from build123d import *

# Parameters (mm, degrees)
SKETCH1_R           = 5
BOSS_EXTRUDE1_DEPTH = 3


with BuildPart() as part:
    # Sketch1 → Boss-Extrude1 (new body)
    with BuildSketch(Plane(origin=(0, 0, 0), x_dir=(1, 0, 0), z_dir=(0, 1, 0))):
        Polygon((3, 10), (0, 10), (0, 0), (4, 0), (4, 3), (14, 3), (14, 0), (22, 0), (22, 3), (28, 3), (28, 0), (36, 0), (36, 3), (46, 3), (46, 0), (50, 0), (50, 10), (47, 10), (47, 20), (50, 20), (50, 30), (47, 30), (47, 40), (50, 40), (50, 50), (47, 50), (47, 60), (50, 60), (50, 70), (47, 70), (47, 80), (50, 80), (50, 90), (47, 90), (47, 100), (50, 100), (50, 110), (47, 110), (47, 120), (3, 120), (3, 110), (0, 110), (0, 100), (3, 100), (3, 90), (0, 90), (0, 80), (3, 80), (3, 70), (0, 70), (0, 60), (3, 60), (3, 50), (0, 50), (0, 40), (3, 40), (3, 30), (0, 30), (0, 20), (3, 20), align=None)
        with Locations(Location((25, 40, 0), (0, 0, 270))):
            Circle(SKETCH1_R, mode=Mode.SUBTRACT)
        with Locations(Location((25, 80, 0), (0, 0, 270))):
            Circle(SKETCH1_R, mode=Mode.SUBTRACT)
    extrude(amount=BOSS_EXTRUDE1_DEPTH)


solid = part.part
Geometry check sheet. Reference: the model listing, model coordinates, mm. A direction names the side the tool comes from. Coordinates: 2 decimals unless noted, no trailing zeros. Write each loop counter-clockwise with the first axis right and the second up, starting at its lowest first coordinate (ties: lowest second). Pieces come first, ordered by that corner, then holes. Notation, with made-up numbers: (70.5, -29) -> (122.5, -29) arc R14 ccw to (122.5, -22) -> close; hole circle Ø2 at (1, 9). An arc over 180 degrees is marked (long way). One line per question, with ' | ' between items.
1. Cross-section at C-C on y = 2.1. State how many separate pieces and enclosed holes the cut face has, and give its area (3 significant figures).
Answers:
separate pieces: 1 | enclosed holes: 2 | area: 5,400 mm²
2. Cross-section at B-B on x = 25. Record the cut outline in (y, z), and give its area (3 significant figures).
Answers:
outline: (0, -120) -> (3, -120) -> (3, -85) -> (0, -85) -> close; (0, -75) -> (3, -75) -> (3, -45) -> (0, -45) -> close; (0, -35) -> (3, -35) -> (3, -3) -> (0, -3) -> close | area: 291 mm²
3. Thickness scan on probe 1 along Z at (x, y) = (43, 2.85); probe 2 along Z at (x, y) = (22.5, 1.3); probe 3 along X at (y, z) = (0.4, -76.5). Record the ranges inside material, lowest first. Write a range as from..to.
Answers:
probe 1: z = -120..-3 | probe 2: z = -120..-84.33, -75.67..-44.33, -35.67..-3 | probe 3: x = 3..21.43, 28.57..47
4. Depth check by flat-ended pin: pin 1 Ø0.9 at (y, z) = (1, -16) entering from +X; pin 2 Ø1.5 at (x, y) = (2, 1) entering from -Z; pin 3 Ø1 at (y, z) = (2, -53.5) entering from -X. Enter the tip coordinate at first touch or a pass-through.
Answers:
pin 1: stops at x = 47 | pin 2: stops at z = -110 | pin 3: stops at x = 3
5. Cross-section at D-D on z = -17. Record the cut outline in (x, y), and give its area (3 significant figures).
Answers:
outline: (3, 0) -> (47, 0) -> (47, 3) -> (3, 3) -> close | area: 132 mm²
6. Set-up check for faces 1 (the flat face through (49, 1, -50)), 2 (the flat face through (14, 1, -2)), 3 (the flat face through (2, 1, -30)), 4 (the cylindrical face through (22, 1, -44)): record each of +Z, -Z, +X, -X, +Y, -Y from which the full face is reachable in a straight line by a thin tool's end or side.
Answers:
face 1: +X, +Y, -Y | face 2: +Z, +Y, -Y | face 3: -X, +Y, -Y | face 4: +Y, -Y
7. Cross-section at A-A on z = -43. Record the cut outline in (x, y), and give its area (3 significant figures).
Answers:
outline: (0, 0) -> (21, 0) -> (21, 3) -> (0, 3) -> close; (29, 0) -> (50, 0) -> (50, 3) -> (29, 3) -> close | area: 126 mm²
8. Draft check along X on faces 5 (the flat face through (46, 1, -2)), 6 (the flat face through (0, 1, -45)), 7 (the flat face through (25, 0, -61)), 8 (the flat face through (50, 1, -5)). Enter one of: +X half, -X half, draft (parallel to the pull), parting line (faces both ways), or undercut.
Answers:
face 5: undercut | face 6: -X half | face 7: draft | face 8: +X half
